Input: dimensioned drawing with shaded views. Units: mm. Origin: part minimum x, y, z. Coordinates: 2 decimals unless noted, no trailing zeros. Write each loop counter-clockwise with the first axis right and the second up, starting at its lowest first coordinate (ties: lowest second). Pieces come first, ordered by that corner, then holes. Notation, with made-up numbers: M -7.5,31 L 2.5,31 A24 ccw 2.5,52 Z; hole C -8,-2 d1. An arc over 180 degrees is marked long. Use one line per item in the form item = value.
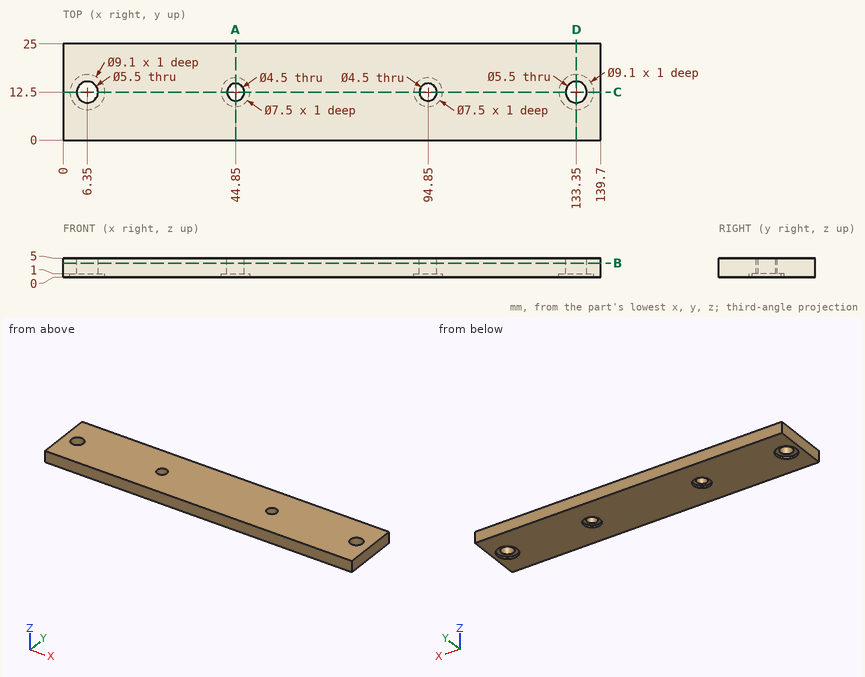
(1) Section query C-C on y = 12.5. State how many separate pieces and enclosed holes the cut face has, plus the area to 3 significant figures.
Computed:
separate_pieces = 5
enclosed_holes = 0
area = 585 mm^2
(2) First-contact query: pin 1 Ø4 at (x, y) = (95.5, 11.5) entering from -Z. Flat tip, straight axial feed; report the tip coordinate or a pass-through.
Computed:
pin_1 = 1
(3) Section query D-D on x = 133.35. Return the cut outline in (y, z).
Computed:
outline = M 0,0 L 7.95,0 L 7.95,1 L 9.75,1 L 9.75,5 L 0,5 Z; M 15.25,1 L 17.05,1 L 17.05,0 L 25,0 L 25,5 L 15.25,5 Z
(4) Section query A-A on x = 44.85. Return the cut outline in (y, z), plus the area to 3 significant figures.
Computed:
outline = M 0,0 L 8.75,0 L 8.75,1 L 10.25,1 L 10.25,5 L 0,5 Z; M 14.75,1 L 16.25,1 L 16.25,0 L 25,0 L 25,5 L 14.75,5 Z
area = 99.5 mm^2
(5) Section query B-B on z = 3.75. Return the cut outline in (x, y).
Computed:
outline = M 0,0 L 139.7,0 L 139.7,25 L 0,25 Z; hole C 6.35,12.5 d5.5; hole C 44.85,12.5 d4.5; hole C 94.85,12.5 d4.5; hole C 133.35,12.5 d5.5
(6) Line query: probe 1 along X at (y, z) = (12.5, 2.2); probe 2 along X at (y, z) = (12.5, 0.2); probe 3 along Y at (x, z) = (133.35, 0.6). Output: solid intervals per line, ascending.
Computed:
probe_1 = 0 to 3.6, 9.1 to 42.6, 47.1 to 92.6, 97.1 to 130.6, 136.1 to 139.7
probe_2 = 0 to 1.8, 10.9 to 41.1, 48.6 to 91.1, 98.6 to 128.8, 137.9 to 139.7
probe_3 = 0 to 7.95, 17.05 to 25
